Geometry check sheet. Reference: drawing and pictorial views, mm from the part's lowest x, y, z. A direction names the side the tool comes from. Round coordinates to 2 decimals unless told otherwise and drop trailing zeros. Loops run counter-clockwise (first coordinate to the right, second up) from the corner with the lowest first, then second, coordinate; pieces in that order, holes last. Notation, with made-up numbers: (57.25, -26.75) - (74.25, -26.75) arc R17 ccw to (74.25, -19.75) - close; hole circle Ø4 at (77, 20.5). An arc over 180 degrees is marked (long way). Answer as CSV lines item,"result". Start each with the question number.
1) Thickness scan on line 1 along X through (y, z) = (29.5, 2.9); line 2 along Y through (x, z) = (10, 2.05); line 3 along X through (y, z) = (21, 0.3). Record the ranges inside material, lowest first.
2) Draft check along Y on the marked faces 1, 2 and 3. Enter one of: released by +Y, released by -Y, zero draft, split by the parting line, or undercut.
3) Cross-section at B-B on x = 10. Record the boundary of the cut face in (y, z).
4) Access from +Z, -Z, +X, -X, +Y, -Y to the whole of each face (thin tool, end or side, straight path). Record for the marked faces 4, 5 and 6.
5) Cross-section at A-A on y = 29.5. Record the boundary of the cut face in (x, z).
6) Depth check by flat-ended pin: P1, Ø0.9, axis at y = 29.5, z = 1.5, coming from the -X side; P2, Ø1.5, axis at y = 28, z = 1, coming from the +X side; P3, Ø0.8, axis at x = 10.5, z = 2, coming from the +Y side; P4, Ø8, axis at x = 2.5, y = 26, coming from the -Z side. Enter the tip coordinate at first touch or a pass-through.
7) Cross-section at D-D on x = 4.5. Record the boundary of the cut face in (y, z) (1 decimal), and give its area (3 significant figures).
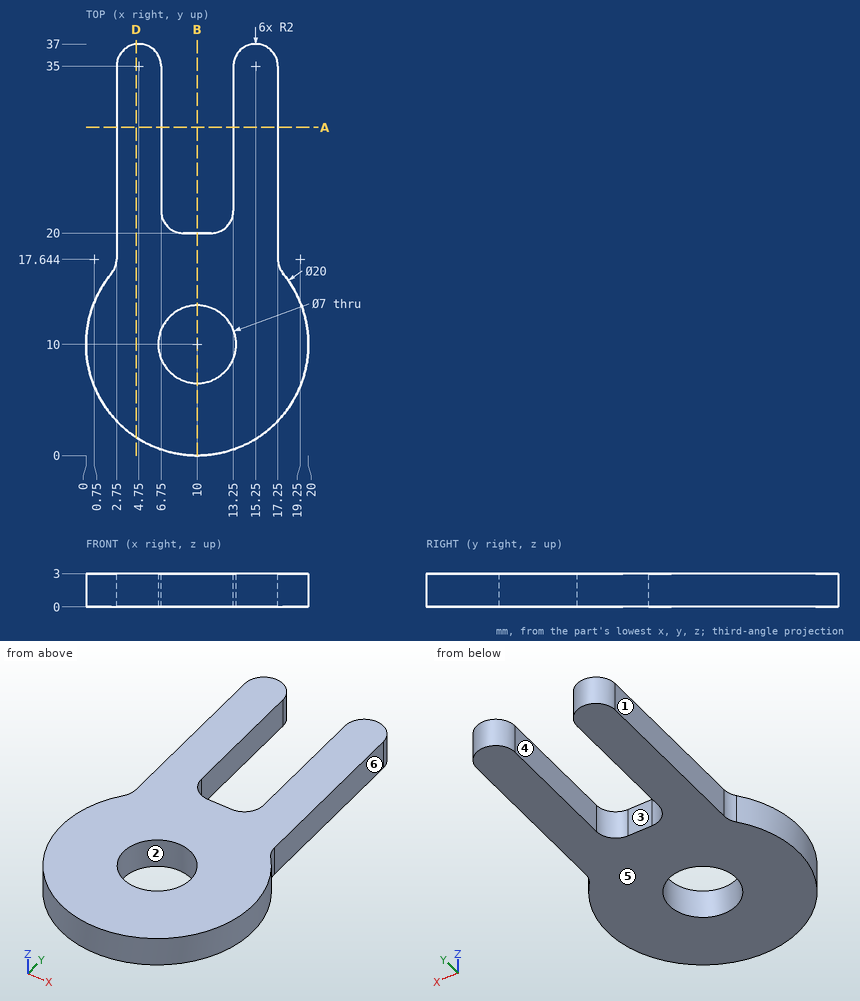
Answer block:
1,line 1,"x = 2.75 to 6.75, 13.25 to 17.25"
1,line 2,"y = 0 to 6.5, 13.5 to 20"
1,line 3,"x = 2.75 to 7.02, 12.98 to 17.25"
2,face 1,"zero draft"
2,face 2,"undercut"
2,face 3,"released by +Y"
3,outline,"(0, 0) - (6.5, 0) - (6.5, 3) - (0, 3) - close; (13.5, 0) - (20, 0) - (20, 3) - (13.5, 3) - close"
4,face 4,"+Z, -Z, +Y"
4,face 5,"-Z, +X, -X, +Y, -Y"
4,face 6,"+Z, -Z, +X, +Y"
5,outline,"(2.75, 0) - (6.75, 0) - (6.75, 3) - (2.75, 3) - close; (13.25, 0) - (17.25, 0) - (17.25, 3) - (13.25, 3) - close"
6,P1,"stops at x = 2.75"
6,P2,"stops at x = 17.25"
6,P3,"stops at y = 20"
6,P4,"stops at z = 0"
7,outline,"(1.6, 0) - (37, 0) - (37, 3) - (1.6, 3) - close"
7,area,"106 mm^2"
